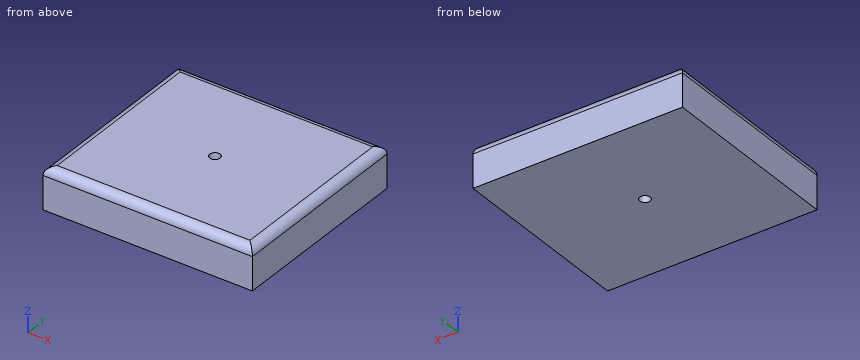
```python
from build123d import *

# Parameters (mm, degrees)
F0_W     = 127.66026
F0_H     = 115.070366
F1_DEPTH = 25.4
F2_R     = 5.08
F4_D     = 6.35


with BuildPart() as f1:
    # F0 (on Top) → F1 (new body)
    with BuildSketch(Plane.XY):
        Rectangle(F0_W, F0_H)
    extrude(amount=F1_DEPTH)

    # F2
    f2_edges = [f1.edges().sort_by_distance(p)[0] for p in [
        (0, -57.535183, 25.4),
        (63.83013, 0, 25.4),
        (0, 57.535183, 25.4),
        (-63.83013, 0, 25.4),
    ]]
    fillet(f2_edges, radius=F2_R)

    # F4 (through all)
    with Locations(Plane.XY.offset(25.4)):
        with Locations((0, 0)):
            Hole(F4_D / 2)


solid = f1.part
```
Model file for the job. Use its own axes, mm. Give positions to 0.01 mm unless a question says otherwise; leave off trailing zeros. Write each loop counter-clockwise with the first axis right and the second up, starting at its lowest first coordinate (ties: lowest second). Pieces come first, ordered by that corner, then holes. Notation, with made-up numbers: (35.25, 82) - (65.25, 82) arc R23 cw to (65.25, 92) - close; hole circle Ø9 at (16, -38.75). An arc over 180 degrees is marked (long way). One line per question, with ' | ' between items. Start each with the question number.
(1) Slice it at A-A on x = 0. Write the cut outline in (y, z) (3 decimals), plus the area to 3 significant figures.
(2) Wall check: line 1 along Y through (x, z) = (0, 8) (3 decimals); line 2 along X through (y, z) = (49.5, 20.75). Give the ranges that are in metal, low to high. Write a range as from..to.
(3) Slice it at B-B on y = 0. Write the cut outline in (x, z) (3 decimals).
(4) Slice it at C-C on z = 22.5. Write the cut outline in (x, y) (3 decimals).
Results below:
1) outline: (-57.535, 0) - (-3.175, 0) - (-3.175, 25.4) - (-52.455, 25.4) arc R5.08 ccw to (-57.535, 20.32) - close; (3.175, 0) - (57.535, 0) - (57.535, 20.32) arc R5.08 ccw to (52.455, 25.4) - (3.175, 25.4) - close | area: 2,750 mm^2
2) line 1: -57.535..-3.175, 3.175..57.535 | line 2: -63.81..63.81
3) outline: (-63.83, 0) - (-3.175, 0) - (-3.175, 25.4) - (-58.75, 25.4) arc R5.08 ccw to (-63.83, 20.32) - close; (3.175, 0) - (63.83, 0) - (63.83, 20.32) arc R5.08 ccw to (58.75, 25.4) - (3.175, 25.4) - close
4) outline: (-63.339, -57.044) - (63.339, -57.044) - (63.339, 57.044) - (-63.339, 57.044) - close; hole circle Ø6.35 at (0, 0)
